Could you check a few things on this model? Use its own coordinates, in mm. Face numbers are marked on the shaded views. A direction names the side the tool comes from. Coordinates: 2 decimals unless noted, no trailing zeros. Order: outer loops, then holes, each group sorted by start corner. A loop starts at its lowest first (then second) coordinate and runs counter-clockwise, first axis right, second up.
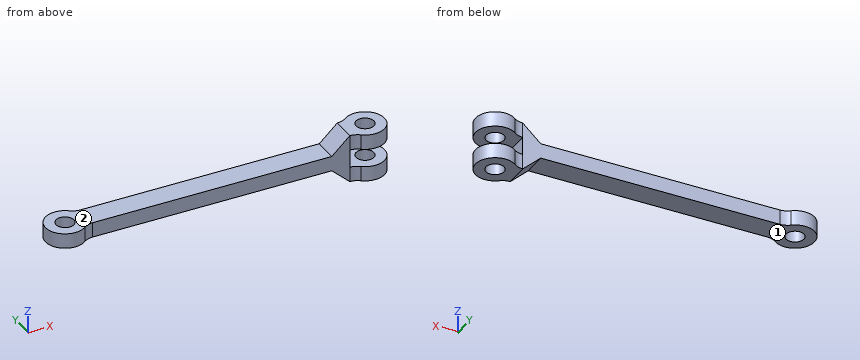
```python
from build123d import *
from build123d.topology import SkipClean

# Parameters (mm, degrees)
SKETCH1_R               = 30
BOSS_EXTRUDE1_DEPTH     = 25
SKETCH3_R               = 30
BOSS_EXTRUDE2_DEPTH     = 80
CUT_EXTRUDE1_DEPTH      = 1074.14957019
CUT_EXTRUDE1_DEPTH_BACK = 1074.14957019
SKETCH4_W               = 136.589105316
SKETCH4_H               = 60


with BuildPart() as part:
    # Sketch1 → Boss-Extrude1 (new, symmetric)
    with BuildSketch(Plane.XY):
        with BuildLine():
            Line((71.589105316, 40), (928.410894684, 40))
            ThreePointArc((928.410894684, 40), (944.895406519, 42.795541847), (959.536592647, 50.869565217))
            ThreePointArc((959.536592647, 50.869565217), (1065, 0), (959.536592647, -50.869565217))
            ThreePointArc((959.536592647, -50.869565217), (944.895406519, -42.795541847), (928.410894684, -40))
            Line((928.410894684, -40), (71.589105316, -40))
            ThreePointArc((71.589105316, -40), (55.104593481, -42.795541847), (40.463407353, -50.869565217))
            ThreePointArc((40.463407353, -50.869565217), (-65, 0), (40.463407353, 50.869565217))
            ThreePointArc((40.463407353, 50.869565217), (55.104593481, 42.795541847), (71.589105316, 40))
        make_face()
        Circle(SKETCH1_R, mode=Mode.SUBTRACT)
        with Locations((1000, 0)):
            Circle(SKETCH1_R, mode=Mode.SUBTRACT)
    extrude(amount=BOSS_EXTRUDE1_DEPTH, both=True)

    # Sketch3 → Boss-Extrude2 (add, symmetric)
    with SkipClean():  # the faces are left unmerged after this step: merging them gives an invalid solid
        with BuildSketch(Plane.XY):
            with BuildLine():
                Line((868.410894684, -40), (928.410894684, -40))
                ThreePointArc((928.410894684, -40), (944.895406519, -42.795541847), (959.536592647, -50.869565217))
                ThreePointArc((959.536592647, -50.869565217), (1065, 0), (959.536592647, 50.869565217))
                ThreePointArc((959.536592647, 50.869565217), (944.895406519, 42.795541847), (928.410894684, 40))
                Line((928.410894684, 40), (868.410894684, 40))
                Line((868.410894684, 40), (868.410894684, -40))
            make_face()
            with Locations((1000, 0)):
                Circle(SKETCH3_R, mode=Mode.SUBTRACT)
        extrude(amount=BOSS_EXTRUDE2_DEPTH, both=True)

    # Sketch4 → Cut-Extrude1 (cut, two sides: drawn at the far end of the back side and taken through both)
    with BuildSketch(Plane(origin=(0, 40, 0), x_dir=(1, 0, 0), z_dir=(0, 1, 0)).offset(-CUT_EXTRUDE1_DEPTH_BACK)):
        Polygon((868.410894684, 25), (928.410894684, 80), (868.410894684, 80), align=None)
        with Locations((996.705447342, 0)):
            Rectangle(SKETCH4_W, SKETCH4_H)
        Polygon((928.410894684, -80), (868.410894684, -80), (868.410894684, -25), align=None)
    extrude(amount=CUT_EXTRUDE1_DEPTH + CUT_EXTRUDE1_DEPTH_BACK, mode=Mode.SUBTRACT)


solid = part.part
```
Item 1: Which directions (+Z, -Z, +X, -X, +Y, -Y) give clear straight access to the entire face, cutting with the end or side of a thin tool? Please do the marked faces 1 and 2.
Item 2: Suppose I cut it at A-A (y = 0). List the corners of the cut face in (x, z) for me.
Item 3: I need wall thicknesses on line 1 (Y direction, x = 1000, z = 41.5); line 2 (Z direction, x = 956, y = -4); line 3 (Z direction, x = 312, y = -24). Which ranges of each line are inside material? Lowest first, please.
Item 4: Suppose I cut it at C-C (x = 1000). List the corners of the cut face in (y, z) for me.
Item 5: For pin 1 Ø5 at (x, y) = (335, -19) entering from -Z; pin 2 Ø1 at (y, z) = (18, 5.5) entering from +X; pin 3 Ø4 at (y, z) = (50.5, -2.5) entering from -X, each with a flat end and sliding along its axis, tell me the tip position at first contact or that it passes through.
Item 6: Suppose I cut it at D-D (z = -4.5). List the corners of the cut face in (x, y) for me, and give its area (3 significant figures).
Item 7: Suppose I cut it at B-B (x = 0). List the corners of the cut face in (y, z) for me, and give its area (3 significant figures).
Geometry results:
1. face 1: -Z, -X, +Y, -Y
1. face 2: +Z, -X, +Y, -Y
2. outline: (-65, -25) - (-30, -25) - (-30, 25) - (-65, 25) - close; (30, -25) - (868.41, -25) - (928.41, -80) - (970, -80) - (970, -30) - (928.41, -30) - (928.41, 30) - (970, 30) - (970, 80) - (928.41, 80) - (868.41, 25) - (30, 25) - close; (1030, -80) - (1065, -80) - (1065, -30) - (1030, -30) - close; (1030, 30) - (1065, 30) - (1065, 80) - (1030, 80) - close
3. line 1: y = -65 to -30, 30 to 65
3. line 2: z = -80 to -30, 30 to 80
3. line 3: z = -25 to 25
4. outline: (-65, -80) - (-30, -80) - (-30, -30) - (-65, -30) - close; (-65, 30) - (-30, 30) - (-30, 80) - (-65, 80) - close; (30, -80) - (65, -80) - (65, -30) - (30, -30) - close; (30, 30) - (65, 30) - (65, 80) - (30, 80) - close
5. pin 1: stops at z = -25
5. pin 2: stops at x = 928.41
5. pin 3: stops at x = -43.28
6. outline: (40.46, -50.87) arc R50 cw to (71.59, -40) - (928.41, -40) - (928.41, 40) - (71.59, 40) arc R50 cw to (40.46, 50.87) arc R65 ccw (long way) to start; hole circle Ø60 at (0, 0)
6. area: 80,000 mm2
7. outline: (-65, -25) - (-30, -25) - (-30, 25) - (-65, 25) - close; (30, -25) - (65, -25) - (65, 25) - (30, 25) - close
7. area: 3,500 mm2
